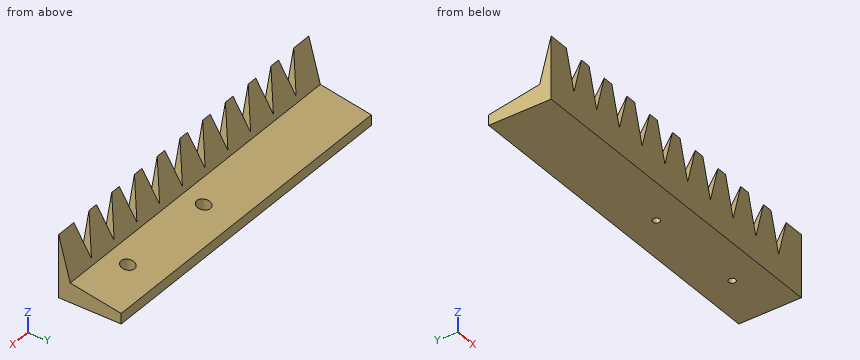
```python
from build123d import *

# Parameters (mm, degrees)
BOSS_EXTRUDE1_DEPTH  = 100
M3_CLEARANCE_HOLE1_D = 3.4
SKETCH4_R            = 3.25
CUT_EXTRUDE1_DEPTH   = 108.964114408
BOSS_EXTRUDE2_DEPTH  = 65
CUT_EXTRUDE2_DEPTH   = 109.627804912
LPATTERN1_COUNT      = 10
LPATTERN1_PITCH      = 15


with BuildPart() as part:
    # Sketch1 → Boss-Extrude1 (new body)
    with BuildSketch(Plane(origin=(0, 0, 0), x_dir=(0, 0, -1), z_dir=(1, 0, 0))):
        Polygon((0, 0), (0, 30), (-5, 30), (-9.312388631, 5.54322876), (-30, 0), align=None)
    extrude(amount=BOSS_EXTRUDE1_DEPTH)

    # M3 Clearance Hole1 (through all)
    with Locations(Plane(origin=(0, 0, 0), x_dir=(-1, 0, 0), z_dir=(0, 0, -1))):
        with Locations((-25, 15), (-75, 15)):
            Hole(M3_CLEARANCE_HOLE1_D / 2)

    # Sketch4 → Cut-Extrude1 (cut, through all)
    with BuildSketch(Plane(origin=(0, 0, 2.5), x_dir=(-1, 0, 0), z_dir=(0, 0, -1))):
        with Locations((-75, 15)):
            Circle(SKETCH4_R)
        with Locations((-25, 15)):
            Circle(SKETCH4_R)
    extrude(amount=-CUT_EXTRUDE1_DEPTH, mode=Mode.SUBTRACT)

    # Sketch6 → Boss-Extrude2 (add)
    with BuildSketch(Plane.ZY):
        Polygon((0, 0), (30, 0), (9.312388631, 5.54322876), (5, 30), (0, 30), align=None)
    extrude(amount=BOSS_EXTRUDE2_DEPTH)

    # Sketch7 → Cut-Extrude2 (cut, symmetric)
    with BuildSketch(Plane(origin=(0, 0, 0), x_dir=(1, 0, 0), z_dir=(0, 1, 0))):
        Polygon((-55, -30), (-50, -12), (-45, -30), align=None)
    cut_extrude2 = extrude(amount=CUT_EXTRUDE2_DEPTH, both=True, mode=Mode.SUBTRACT)

    # LPattern1: Cut-Extrude2 ×10
    with Locations(*[(i * LPATTERN1_PITCH, 0, 0) for i in range(1, LPATTERN1_COUNT)]):
        add(cut_extrude2, mode=Mode.SUBTRACT)


solid = part.part
```
Can you work these out from the model? Positions are in its coordinate system, mm. Give positions to 0.01 mm unless a question says otherwise; leave off trailing zeros. Loops run counter-clockwise (first coordinate to the right, second up) from the corner with the lowest first, then second, coordinate; pieces in that order, holes last. Notation, with made-up numbers: M -7,-30 L 27,-30 A20 cw 27,-23 Z; hole C 47,52 d8. An arc over 180 degrees is marked long. One line per item, written item: value.
(1) Suppose I cut it at A-A on y = 15. List the corners of the cut face in (x, z) for me.
Returned:
outline: M -65,0 L 23.3,0 L 23.3,2.5 L 21.75,2.5 L 21.75,7.64 L -65,7.64 Z; M 26.7,0 L 73.3,0 L 73.3,2.5 L 71.75,2.5 L 71.75,7.64 L 28.25,7.64 L 28.25,2.5 L 26.7,2.5 Z; M 76.7,0 L 100,0 L 100,7.64 L 78.25,7.64 L 78.25,2.5 L 76.7,2.5 Z
(2) Suppose I cut it at C-C on z = 15. Count the separate pieces of the cut face and the enclosed holes in it, plus the area to 3 significant figures.
Returned:
separate pieces: 11
enclosed holes: 0
area: 596 mm^2
(3) Will these pins go through, and if not, where does the flat tip stop? pin 1 (4 mm diameter, centred on x = -7, y = 8, fed in from +Z); pin 2 (2 mm diameter, centred on x = 26, y = 16, fed in from +Z); pin 3 (4 mm diameter, centred on x = 35.5, y = 23.5, fed in from +Z).
Returned:
pin 1: z = 9.23
pin 2: z = 2.5
pin 3: z = 6.5
(4) Suppose I cut it at B-B on x = 3. List the corners of the cut face in (y, z) for me.
Returned:
outline: M 0,0 L 30,0 L 30,5 L 5.54,9.31 L 0,30 Z
(5) I need wall thicknesses on line 1 (X direction, y = 15, z = 5); line 2 (Y direction, x = 75, z = 3.95); line 3 (Z direction, x = 22, y = 14). Which ranges of each line are inside material? Lowest first, please.
Returned:
line 1: -65 to 21.75, 28.25 to 71.75, 78.25 to 100
line 2: 0 to 11.75, 18.25 to 30
line 3: 0 to 2.5
